Geometry check sheet. Reference: drawing and pictorial views, mm from the part's lowest x, y, z. A direction names the side the tool comes from. Give positions to 0.01 mm unless a question says otherwise; leave off trailing zeros. Write each loop counter-clockwise with the first axis right and the second up, starting at its lowest first coordinate (ties: lowest second). Pieces come first, ordered by that corner, then holes. Notation, with made-up numbers: M 40,41 L 77,41 A25 cw 77,78 Z; hole C 65,20.5 d9. An arc over 180 degrees is marked long. Write item = value, one per line. Start each with the question number.
1) Cross-section at C-C, the plane y = 12.7. Record the cut outline in (x, z), plus the area to 3 significant figures.
2) Go/stop test with flat-tipped pins: pin 1 (12.5 mm diameter, centred on y = 16.5, z = 15.5, fed in from -X); pin 2 (6.5 mm diameter, centred on x = 43, y = 12.5, fed in from +Z); pin 3 (12 mm diameter, centred on y = 16.5, z = 12, fed in from +X). Record where each tip stops, or that it passes through.
3) Cross-section at B-B, the plane z = 15.24. Record the cut outline in (x, y).
4) Access from +Z, -Z, +X, -X, +Y, -Y to the whole of each face (thin tool, end or side, straight path). Record for the marked faces 1, 2, 3 and 4.
5) Scan lines: line 1 along X through (y, z) = (19.25, 5); line 2 along Y through (x, z) = (36, 15.24); line 3 along Z through (x, y) = (48.5, 5.5). Record each from-to range of solid material in increasing order. Write a range as [from, to].
6) Cross-section at A-A, the plane z = 5. Record the cut outline in (x, y), plus the area to 3 significant figures.
7) Cross-section at D-D, the plane x = 17.5. Record the cut outline in (y, z), plus the area to 3 significant figures.
8) Mould release check, pull along X, two halves, no side actions. Record for the marked faces 5, 6 and 7: released by +X, released by -X, zero draft, split by the parting line, or undercut.
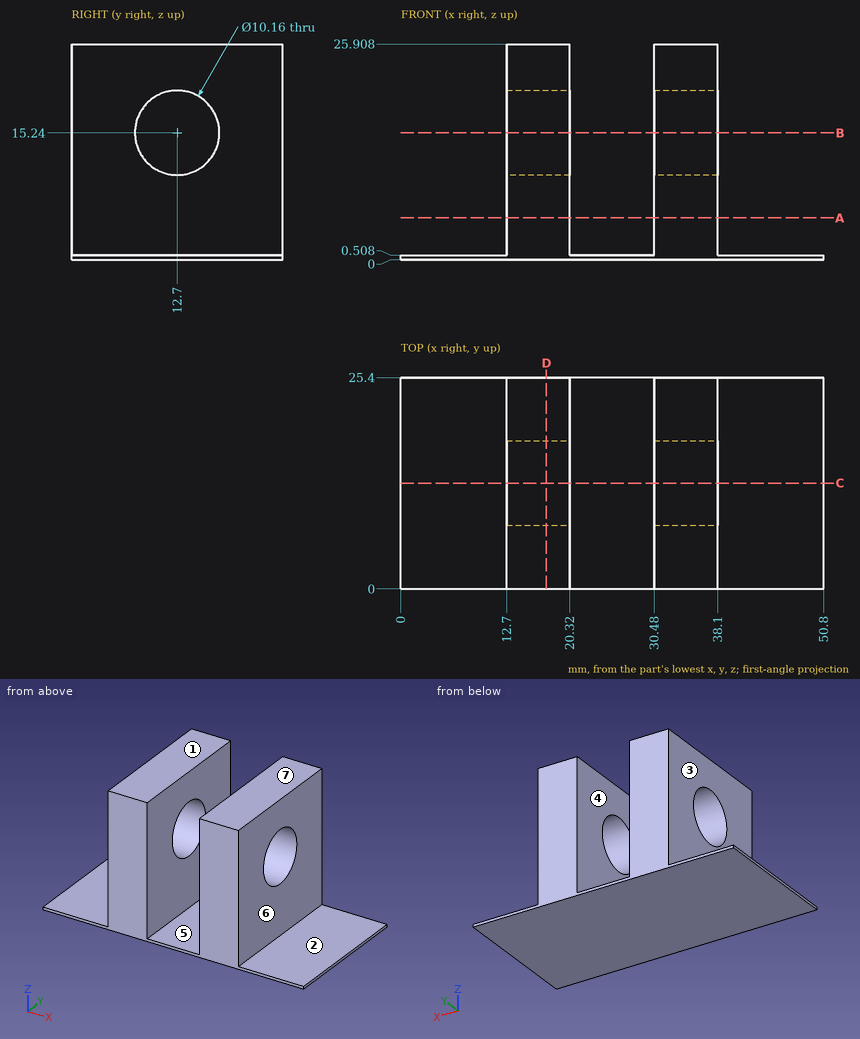
Reply:
q1.outline = M 0,0 L 50.8,0 L 50.8,0.51 L 38.1,0.51 L 38.1,10.16 L 30.48,10.16 L 30.48,0.51 L 20.32,0.51 L 20.32,10.16 L 12.7,10.16 L 12.7,0.51 L 0,0.51 Z; M 12.7,20.32 L 20.32,20.32 L 20.32,25.91 L 12.7,25.91 Z; M 30.48,20.32 L 38.1,20.32 L 38.1,25.91 L 30.48,25.91 Z
q1.area = 258 mm2
q2.pin_1 = 12.7
q2.pin_2 = 0.51
q2.pin_3 = 38.1
q3.outline = M 12.7,0 L 20.32,0 L 20.32,7.62 L 12.7,7.62 Z; M 12.7,17.78 L 20.32,17.78 L 20.32,25.4 L 12.7,25.4 Z; M 30.48,0 L 38.1,0 L 38.1,7.62 L 30.48,7.62 Z; M 30.48,17.78 L 38.1,17.78 L 38.1,25.4 L 30.48,25.4 Z
q4.face_1 = +Z, +X, -X, +Y, -Y
q4.face_2 = +Z, +X, +Y, -Y
q4.face_3 = +Z, -X, +Y, -Y
q4.face_4 = +Z, +Y, -Y
q5.line_1 = [12.7, 20.32], [30.48, 38.1]
q5.line_2 = [0, 7.62], [17.78, 25.4]
q5.line_3 = [0, 0.51]
q6.outline = M 12.7,0 L 20.32,0 L 20.32,25.4 L 12.7,25.4 Z; M 30.48,0 L 38.1,0 L 38.1,25.4 L 30.48,25.4 Z
q6.area = 387 mm2
q7.outline = M 0,0 L 25.4,0 L 25.4,25.91 L 0,25.91 Z; hole C 12.7,15.24 d10.16
q7.area = 577 mm2
q8.face_5 = undercut
q8.face_6 = released by +X
q8.face_7 = zero draft
